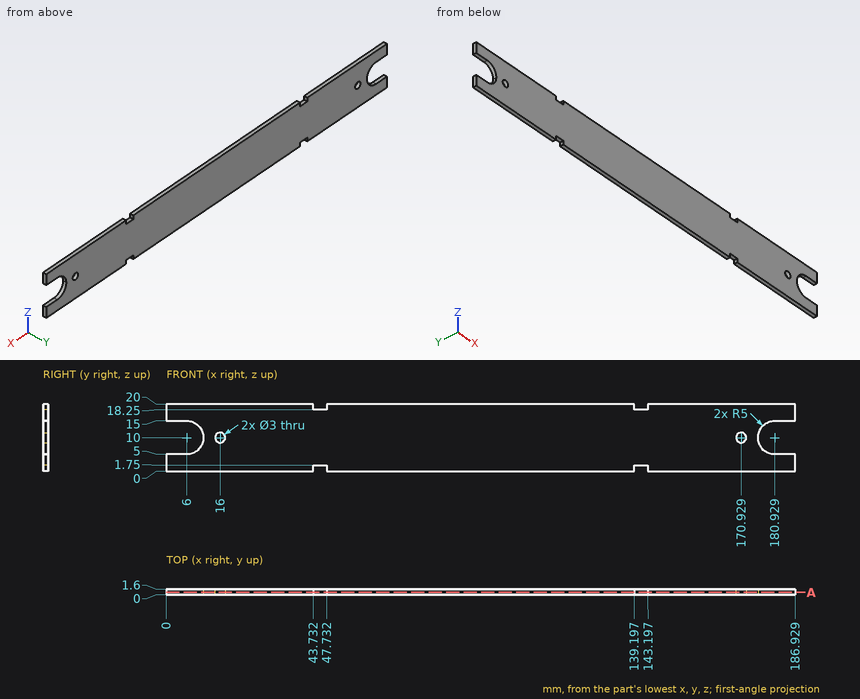
Check sheet for the drawn part. Datum: minimum x, y, z corner. Units: mm. Round coordinates to 2 decimals unless told otherwise and drop trailing zeros. Write each question's results on one line, items separated by ' | '.
1) Gauge pin test, flat ends, axial feed: P1, Ø0.8, axis at x = 141, y = 0.5, coming from the -Z side; P2, Ø0.8, axis at x = 141.5, y = 0.5, coming from the +Z side; P3, Ø2, axis at x = 164, z = 10.5, coming from the -Y side. Record the tip position at first contact, or that the pin passes through.
Checks:
P1: stops at z = 1.75 | P2: stops at z = 18.25 | P3: stops at y = 0
2) Scan lines: L1, parallel to X at y = 0.55, z = 19; L2, parallel to X at y = 0.8, z = 11.25; L3, parallel to X at y = 0.2, z = 7.5. Record each from-to range of solid material in increasing order. Write a range as from..to.
Checks:
L1: x = 0..43.73, 47.73..139.2, 143.2..186.93 | L2: x = 10.84..15.17, 16.83..170.1, 171.76..176.09 | L3: x = 10.33..176.6
3) Section check A-A on y = 0.7. State how many separate pieces and enclosed holes the cut face has, then the cut area to 3 significant figures.
Checks:
separate pieces: 1 | enclosed holes: 2 | area: 3,500 mm2
